Geometry: final body of the model. Coordinates: model frame, mm. Coordinates: 2 decimals unless noted, no trailing zeros. Write each loop counter-clockwise with the first axis right and the second up, starting at its lowest first coordinate (ties: lowest second). Pieces come first, ordered by that corner, then holes.
from build123d import *

# Parameters (mm, degrees)
SKETCH1_R           = 1.016
SKETCH1_R_2         = 3.7592
BOSS_EXTRUDE1_DEPTH = 1.5875


with BuildPart() as part:
    # Sketch1 → Boss-Extrude1 (new body)
    with BuildSketch(Plane(origin=(0, 0, 0), x_dir=(0, 0, -1), z_dir=(1, 0, 0))):
        with BuildLine():
            Line((83.936378182, 3.55409512), (0.206155636, 6.29582564))
            ThreePointArc((0.206155636, 6.29582564), (-6.2992, 9e-09), (0.206155618, -6.295825641))
            Line((0.206155618, -6.295825641), (83.936378182, -3.55409512))
            ThreePointArc((83.936378182, -3.55409512), (87.376, 0), (83.936378182, 3.55409512))
        make_face()
        with BuildLine():
            ThreePointArc((4.654808766, -4.244134305), (6.2992, 0), (4.654808766, 4.244134305))
            Line((4.654808766, 4.244134305), (80.726222273, 1.753190057))
            ThreePointArc((80.726222273, 1.753190057), (80.264, 0), (80.726222273, -1.753190057))
            Line((80.726222273, -1.753190057), (4.654808766, -4.244134305))
        make_face(mode=Mode.SUBTRACT)
        with Locations((83.82, 0)):
            Circle(SKETCH1_R, mode=Mode.SUBTRACT)
        Circle(SKETCH1_R_2, mode=Mode.SUBTRACT)
    extrude(amount=BOSS_EXTRUDE1_DEPTH)


solid = part.part
Item 1: Pull-direction query (Z, two-part tool) for faces 1 (the flat face through (0, 4, -37)), 2 (the cylindrical face through (0.783, -0.077, -87.375)), 3 (the cylindrical face through (0.78, -3.67, 0.81)); classes: released by +Z, released by -Z, zero draft, split by the parting line, or undercut.
Derived:
face 1: zero draft
face 2: released by -Z
face 3: undercut
Item 2: Section A-A, the plane y = 0. Output: boundary loops of the cut face in (x, z), plus the area to 3 significant figures.
Derived:
outline: (0, -87.38) - (1.59, -87.38) - (1.59, -84.84) - (0, -84.84) - close; (0, -82.8) - (1.59, -82.8) - (1.59, -80.26) - (0, -80.26) - close; (0, -6.3) - (1.59, -6.3) - (1.59, -3.76) - (0, -3.76) - close; (0, 3.76) - (1.59, 3.76) - (1.59, 6.3) - (0, 6.3) - close
area: 16.1 mm2
Item 3: Section C-C, the plane z = -52. Output: boundary loops of the cut face in (x, y).
Derived:
outline: (0, -4.6) - (1.59, -4.6) - (1.59, -2.69) - (0, -2.69) - close; (0, 2.69) - (1.59, 2.69) - (1.59, 4.6) - (0, 4.6) - close
Item 4: Pin query (flat end, axial travel): pin 1 (3 mm diameter, centred on y = 1, z = -24.5, fed in from -X). Return the tip coordinate at first contact, or that it passes through.
Derived:
pin 1: passes through
Item 5: Material intervals for probe 1 along Y at (x, z) = (1.1, -83.82); probe 2 along Y at (x, z) = (1.2, -5.5); probe 3 along Y at (x, z) = (0.5, 0), sorted ascending.
Derived:
probe 1: y = -3.56 to -1.02, 1.02 to 3.56
probe 2: y = -6.12 to -4.22, -3.07 to 3.07, 4.22 to 6.12
probe 3: y = -6.3 to -3.76, 3.76 to 6.3
Item 6: Section B-B, the plane x = 0.3. Output: boundary loops of the cut face in (y, z).
Derived:
outline: (-6.3, -0.21) - (-3.55, -83.94) arc R3.56 ccw to (3.55, -83.94) - (6.3, -0.21) arc R6.3 ccw (long way) to start; hole (-4.24, -4.65) - (-1.75, -80.73) arc R3.56 cw to (1.75, -80.73) - (4.24, -4.65) arc R6.3 cw to start; hole circle Ø7.52 at (0, 0); hole circle Ø2.03 at (0, -83.82)
